```python
from build123d import *

# Parameters (mm, degrees)
SKETCH1_R           = 1.25
SKETCH1_W           = 11.8
SKETCH1_H           = 22.5
BOSS_EXTRUDE1_DEPTH = 2


with BuildPart() as part:
    # Sketch1 → Boss-Extrude1 (new body)
    with BuildSketch(Plane.XY):
        with BuildLine():
            ThreePointArc((6.057454149, 24.255045851), (0, 25), (-6.057454149, 24.255045851))
            ThreePointArc((-6.057454149, 24.255045851), (-10.281376502, 23.819659541), (-14.458061439, 24.585416821))
            ThreePointArc((-14.458061439, 24.585416821), (-22.656854249, 22.656854249), (-24.585416821, 14.458061439))
            ThreePointArc((-24.585416821, 14.458061439), (-23.819659541, 10.281376502), (-24.255045851, 6.057454149))
            ThreePointArc((-24.255045851, 6.057454149), (-25, 0), (-24.255045851, -6.057454149))
            ThreePointArc((-24.255045851, -6.057454149), (-23.819659541, -10.281376502), (-24.585416821, -14.458061439))
            ThreePointArc((-24.585416821, -14.458061439), (-22.656854249, -22.656854249), (-14.458061439, -24.585416821))
            ThreePointArc((-14.458061439, -24.585416821), (-10.281376502, -23.819659541), (-6.057454149, -24.255045851))
            ThreePointArc((-6.057454149, -24.255045851), (0, -25), (6.057454149, -24.255045851))
            ThreePointArc((6.057454149, -24.255045851), (10.281376502, -23.819659541), (14.458061439, -24.585416821))
            ThreePointArc((14.458061439, -24.585416821), (22.656854249, -22.656854249), (24.585416821, -14.458061439))
            ThreePointArc((24.585416821, -14.458061439), (23.819659541, -10.281376502), (24.255045851, -6.057454149))
            ThreePointArc((24.255045851, -6.057454149), (25, 0), (24.255045851, 6.057454149))
            ThreePointArc((24.255045851, 6.057454149), (23.819659541, 10.281376502), (24.585416821, 14.458061439))
            ThreePointArc((24.585416821, 14.458061439), (22.656854249, 22.656854249), (14.458061439, 24.585416821))
            ThreePointArc((14.458061439, 24.585416821), (10.281376502, 23.819659541), (6.057454149, 24.255045851))
        make_face()
        with Locations((0, 13.65)):
            Circle(SKETCH1_R, mode=Mode.SUBTRACT)
        with Locations(Location((0, -13.65, 0), (0, 0, 180))):
            Circle(SKETCH1_R, mode=Mode.SUBTRACT)
        with BuildLine():
            Line((1.3, -18.65), (-1.3, -18.65))
            ThreePointArc((-1.3, -18.65), (-1.794974747, -18.855025253), (-2, -19.35))
            Line((-2, -19.35), (-2, -19.45))
            ThreePointArc((-2, -19.45), (-1.794974747, -19.944974747), (-1.3, -20.15))
            Line((-1.3, -20.15), (1.3, -20.15))
            ThreePointArc((1.3, -20.15), (1.794974747, -19.944974747), (2, -19.45))
            Line((2, -19.45), (2, -19.35))
            ThreePointArc((2, -19.35), (1.794974747, -18.855025253), (1.3, -18.65))
        make_face(mode=Mode.SUBTRACT)
        Rectangle(SKETCH1_W, SKETCH1_H, mode=Mode.SUBTRACT)
        Polygon((-12.02081528, 10.606601718), (-10.606601718, 12.02081528), (-15.556349186, 16.970562748), (-16.970562748, 15.556349186), align=None, mode=Mode.SUBTRACT)
        Polygon((10.606601718, 12.02081528), (15.556349186, 16.970562748), (16.970562748, 15.556349186), (12.02081528, 10.606601718), align=None, mode=Mode.SUBTRACT)
        Polygon((12.02081528, -10.606601718), (10.606601718, -12.02081528), (15.556349186, -16.970562748), (16.970562748, -15.556349186), align=None, mode=Mode.SUBTRACT)
        Polygon((-16.970562748, -15.556349186), (-12.02081528, -10.606601718), (-10.606601718, -12.02081528), (-15.556349186, -16.970562748), align=None, mode=Mode.SUBTRACT)
    extrude(amount=BOSS_EXTRUDE1_DEPTH)


solid = part.part
```
Geometry: final body of the model. Coordinates: model frame, mm. A direction names the side the tool comes from. Round coordinates to 2 decimals unless told otherwise and drop trailing zeros. Write each loop counter-clockwise with the first axis right and the second up, starting at its lowest first coordinate (ties: lowest second). Pieces come first, ordered by that corner, then holes.
Item 1: Section query B-B (y = 0). Return loops of the section in (x, z).
Item 2: Section query D-D (y = -13.65). Return loops of the section in (x, z).
Item 3: Section query C-C (z = 0.9). Give the number of separate pieces and of enclosed holes in the cut face, plus the area to 3 significant figures.
Item 4: Section query A-A (x = 0). Return loops of the section in (y, z).
Item 5: Material intervals for L1, parallel to Y at x = 0, z = 0.4; L2, parallel to X at y = -4.5, z = 1.2; L3, parallel to X at y = -13.65, z = 0.55, sorted ascending.
Item 6: Mould query, pull axis X, two halves, no side actions, for faces 1 (the face through (25, 0, 1)), 2 (the face through (-16.254, -16.273, 0.986)), 3 (the face through (-23.817, -10.222, 0.986)), 4 (the face through (16.254, -16.273, 0.986)). Classes: +X half, -X half, draft (parallel to the pull), parting line (faces both ways), or undercut.
Item 7: Pin query (flat end, axial travel): P1, Ø1, axis at x = -0.5, z = 0.5, coming from the -Y side; P2, Ø1, axis at y = 0.5, z = 1, coming from the -X side. Return the tip coordinate at first contact, or that it passes through.
Item 8: Set-up query: faces 5 (the face through (0, -18.65, 1)), 6 (the face through (23.817, 10.222, 0.986)). Return all of +Z, -Z, +X, -X, +Y, -Y with unobstructed straight access to the full face (end or side cutting, diameter ignored); none if empty.
Completed:
1. outline: (-25, 0) - (-5.9, 0) - (-5.9, 2) - (-25, 2) - close; (5.9, 0) - (25, 0) - (25, 2) - (5.9, 2) - close
2. outline: (-24.34, 0) - (-15.06, 0) - (-15.06, 2) - (-24.34, 2) - close; (-12.24, 0) - (-1.25, 0) - (-1.25, 2) - (-12.24, 2) - close; (1.25, 0) - (12.24, 0) - (12.24, 2) - (1.25, 2) - close; (15.06, 0) - (24.34, 0) - (24.34, 2) - (15.06, 2) - close
3. separate pieces: 1
3. enclosed holes: 8
3. area: 2,030 mm2
4. outline: (-25, 0) - (-20.15, 0) - (-20.15, 2) - (-25, 2) - close; (-18.65, 0) - (-14.9, 0) - (-14.9, 2) - (-18.65, 2) - close; (-12.4, 0) - (-11.25, 0) - (-11.25, 2) - (-12.4, 2) - close; (11.25, 0) - (12.4, 0) - (12.4, 2) - (11.25, 2) - close; (14.9, 0) - (25, 0) - (25, 2) - (14.9, 2) - close
5. L1: y = -25 to -20.15, -18.65 to -14.9, -12.4 to -11.25, 11.25 to 12.4, 14.9 to 25
5. L2: x = -24.59 to -5.9, 5.9 to 24.59
5. L3: x = -24.34 to -15.06, -12.24 to -1.25, 1.25 to 12.24, 15.06 to 24.34
6. face 1: +X half
6. face 2: undercut
6. face 3: -X half
6. face 4: undercut
7. P1: stops at y = -25
7. P2: stops at x = -25
8. face 5: +Z, -Z
8. face 6: +Z, -Z, +X
